```python
from build123d import *

# Parameters (mm, degrees)
SKETCH1_W            = 9.7
SKETCH1_H            = 4.4
BOSS_EXTRUDE1_DEPTH  = 0.42
FILLET1_R            = 1
FILLET2_R            = 1
FILLET3_R            = 1
FILLET4_R            = 1
BOSS_EXTRUDE2_DEPTH  = 0.04
BOSS_EXTRUDE3_DEPTH  = 0.04
BOSS_EXTRUDE4_DEPTH  = 0.04
BOSS_EXTRUDE5_DEPTH  = 0.04
BOSS_EXTRUDE6_DEPTH  = 0.04
BOSS_EXTRUDE7_DEPTH  = 0.04
BOSS_EXTRUDE8_DEPTH  = 0.04
BOSS_EXTRUDE9_DEPTH  = 0.04
BOSS_EXTRUDE10_DEPTH = 0.04
SKETCH11_W           = 0.5
SKETCH11_H           = 1
BOSS_EXTRUDE11_DEPTH = 0.04
SKETCH12_W           = 0.5
SKETCH12_H           = 1
BOSS_EXTRUDE12_DEPTH = 0.04
BOSS_EXTRUDE13_DEPTH = 0.025
HOLE1_D              = 0.3
HOLE2_D              = 0.3
HOLE3_D              = 0.3
CHAMFER1_SIZE        = 0.1
CHAMFER2_SIZE        = 0.05
CHAMFER3_SIZE        = 0.1
CHAMFER4_SIZE        = 0.05
CHAMFER5_SIZE        = 0.1
CHAMFER6_SIZE        = 0.1
CHAMFER7_SIZE        = 0.05
CHAMFER8_SIZE        = 0.05


with BuildPart() as part:
    # Sketch1 → Boss-Extrude1 (new body)
    with BuildSketch(Plane.XY):
        with Locations((4.849999999, 2.20000002)):
            Rectangle(SKETCH1_W, SKETCH1_H)
    extrude(amount=-BOSS_EXTRUDE1_DEPTH)

    # Fillet1
    fillet1_edges = [part.edges().sort_by_distance(p)[0] for p in [
        (-1e-09, 2e-08, -0.21),
    ]]
    fillet(fillet1_edges, radius=FILLET1_R)

    # Fillet2
    fillet2_edges = [part.edges().sort_by_distance(p)[0] for p in [
        (-1e-09, 4.40000002, -0.21),
    ]]
    fillet(fillet2_edges, radius=FILLET2_R)

    # Fillet3
    fillet3_edges = [part.edges().sort_by_distance(p)[0] for p in [
        (9.699999999, 2e-08, -0.21),
    ]]
    fillet(fillet3_edges, radius=FILLET3_R)

    # Fillet4
    fillet4_edges = [part.edges().sort_by_distance(p)[0] for p in [
        (9.699999999, 4.40000002, -0.21),
    ]]
    fillet(fillet4_edges, radius=FILLET4_R)

    # Sketch2 → Boss-Extrude2 (add)
    with BuildSketch(Plane.XY):
        Polygon((3.691646515, 0.405675456), (4.19162877, 0.405675456), (4.19162877, 0.255675455), (5.553515055, 0.255675455), (5.553515055, 0.45000002), (5.853515055, 0.45000002), (5.853515055, 0.05000002), (5.553515055, 0.05000002), (5.553515055, 0.105675455), (4.04162877, 0.105675455), (4.04162877, 0.255675455), (2.69162877, 0.255675455), (2.69162877, 1.625675455), (3.54162877, 1.625675455), (3.54162877, 2.031926109), (2.082430938, 2.031926109), (2.082430938, 2.631926109), (2.432448683, 2.631926109), (2.432448683, 2.97790002), (2.082448683, 2.97790002), (2.082448683, 3.57790002), (2.582448683, 3.57790002), (2.582448683, 2.181926109), (3.691646515, 2.181926109), align=None)
    extrude(amount=BOSS_EXTRUDE2_DEPTH)

    # Sketch3 → Boss-Extrude3 (add)
    with BuildSketch(Plane.XY):
        Polygon((6.356700213, 0.05000002), (6.056700213, 0.05000002), (6.056700213, 0.45000002), (6.356700213, 0.45000002), (6.356700213, 0.25000002), (7.899307242, 0.25000002), (7.899307242, 1.334176783), (7.549307242, 1.334176783), (7.549307242, 2.97790002), (6.425655767, 2.97790002), (6.425655767, 3.97790002), (6.925655767, 3.97790002), (6.925655767, 3.12790002), (7.699307242, 3.12790002), (7.699307242, 1.484176783), (9.269307242, 1.484176783), (9.269307242, 0.484176783), (8.049307242, 0.484176783), (8.049307242, 0.10000002), (6.356700213, 0.10000002), align=None)
    extrude(amount=BOSS_EXTRUDE3_DEPTH)

    # Sketch4 → Boss-Extrude4 (add)
    with BuildSketch(Plane.XY):
        Polygon((1.148250377, 3.831121862), (1.148250377, 3.381121862), (1.398250377, 3.381121862), (1.448250377, 3.431121862), (1.448250377, 3.481121862), (1.548250377, 3.481121862), (1.548250377, 3.381121862), (1.448250377, 3.281121862), (1.048250377, 3.281121862), (1.048250377, 3.931121862), (1.448250377, 3.931121862), (1.548250377, 3.831121862), (1.548250377, 3.731121862), (1.448250377, 3.731121862), (1.448250377, 3.781121862), (1.398250377, 3.831121862), align=None)
    extrude(amount=BOSS_EXTRUDE4_DEPTH)

    # Sketch5 → Boss-Extrude5 (add)
    with BuildSketch(Plane.XY):
        Polygon((0.417468966, 3.281121862), (0.417468966, 3.381121862), (0.467468966, 3.381121862), (0.467468966, 3.831121862), (0.417468966, 3.831121862), (0.417468966, 3.931121862), (0.917468966, 3.931121862), (0.917468966, 3.643621862), (0.817468966, 3.643621862), (0.817468966, 3.831121862), (0.567468966, 3.831121862), (0.567468966, 3.381121862), (0.817468966, 3.381121862), (0.817468966, 3.568621862), (0.917468966, 3.568621862), (0.917468966, 3.281121862), align=None)
    extrude(amount=BOSS_EXTRUDE5_DEPTH)

    # Sketch6 → Boss-Extrude6 (add)
    with BuildSketch(Plane.XY):
        Polygon((5.349999999, 0.385416863), (5.049999999, 0.385416863), (5.049999999, 0.785416863), (5.199999999, 0.785416863), (5.199999999, 1.246726542), (4.349999999, 1.246726542), (4.349999999, 2.616726542), (4.869837207, 2.616726542), (4.869837207, 2.97790002), (4.519837207, 2.97790002), (4.519837207, 3.97790002), (5.019837207, 3.97790002), (5.019837207, 2.616726542), (5.349999999, 2.616726542), align=None)
    extrude(amount=BOSS_EXTRUDE6_DEPTH)

    # Sketch7 → Boss-Extrude7 (add)
    with BuildSketch(Plane.XY):
        Polygon((1.691646515, 1.625675456), (1.691646515, 0.255675456), (0.691646515, 0.255675456), (0.691646515, 2.031926109), (0.241646515, 2.031926109), (0.241646515, 2.631926109), (0.841646515, 2.631926109), (0.841646515, 2.181926109), (1.122933895, 2.181926109), (1.122933895, 2.631926109), (1.622933895, 2.631926109), (1.622933895, 2.031926109), (0.841646515, 2.031926109), (0.841646515, 1.625675456), align=None)
    extrude(amount=BOSS_EXTRUDE7_DEPTH)

    # Sketch8 → Boss-Extrude8 (add)
    with BuildSketch(Plane.XY):
        Polygon((3.54196347, 3.57790002), (3.54196347, 3.12790002), (3.884837207, 3.12790002), (3.884837207, 3.97790002), (4.384819462, 3.97790002), (4.384819462, 2.97790002), (3.041945725, 2.97790002), (3.041945725, 3.57790002), align=None)
    extrude(amount=BOSS_EXTRUDE8_DEPTH)

    # Sketch9 → Boss-Extrude9 (add)
    with BuildSketch(Plane.XY):
        Polygon((6.749999999, 1.088728228), (7.183722976, 1.088728228), (7.183722976, 1.246726542), (6.349999999, 1.246726542), (6.349999999, 2.616726542), (7.349999999, 2.616726542), (7.349999999, 0.488728228), (6.749999999, 0.488728228), align=None)
    extrude(amount=BOSS_EXTRUDE9_DEPTH)

    # Sketch10 → Boss-Extrude10 (add)
    with BuildSketch(Plane.XY):
        Polygon((8.499307242, 3.667992872), (8.053251319, 3.667992872), (8.053251319, 3.484176783), (9.269307242, 3.484176783), (9.269307242, 2.484176783), (7.899307242, 2.484176783), (7.899307242, 4.267992872), (8.499307242, 4.267992872), align=None)
    extrude(amount=BOSS_EXTRUDE10_DEPTH)

    # Sketch11 → Boss-Extrude11 (add)
    with BuildSketch(Plane.XY):
        with Locations((5.404837207, 3.47790002)):
            Rectangle(SKETCH11_W, SKETCH11_H)
    extrude(amount=BOSS_EXTRUDE11_DEPTH)

    # Sketch12 → Boss-Extrude12 (add)
    with BuildSketch(Plane.XY):
        with Locations((6.040655767, 3.47790002)):
            Rectangle(SKETCH12_W, SKETCH12_H)
    extrude(amount=BOSS_EXTRUDE12_DEPTH)

    # Sketch19 → Boss-Extrude13 (add)
    with BuildSketch(Plane(origin=(0, 0, -0.42), x_dir=(-1, 0, 0), z_dir=(0, 0, -1))):
        with BuildLine():
            Line((-0.999999999, 4.30000002), (-8.699999999, 4.30000002))
            ThreePointArc((-8.699999999, 4.30000002), (-9.336396102, 4.036396123), (-9.599999999, 3.40000002))
            Line((-9.599999999, 3.40000002), (-9.599999999, 1.00000002))
            ThreePointArc((-9.599999999, 1.00000002), (-9.336396102, 0.363603917), (-8.699999999, 0.10000002))
            Line((-8.699999999, 0.10000002), (-0.999999999, 0.10000002))
            ThreePointArc((-0.999999999, 0.10000002), (-0.363603896, 0.363603917), (-0.099999999, 1.00000002))
            Line((-0.099999999, 1.00000002), (-0.099999999, 3.40000002))
            ThreePointArc((-0.099999999, 3.40000002), (-0.363603896, 4.036396123), (-0.999999999, 4.30000002))
        make_face()
    extrude(amount=BOSS_EXTRUDE13_DEPTH)

    # Hole1 (through all)
    with Locations(Plane.XY.offset(0.04)):
        with Locations((8.199307242, 3.967992872)):
            Hole(HOLE1_D / 2)

    # Hole2 (through all)
    with Locations(Plane.XY.offset(0.04)):
        with Locations((7.049999999, 0.788728228)):
            Hole(HOLE2_D / 2)

    # Hole3 (through all)
    with Locations(Plane.XY.offset(0.04)):
        with Locations((0.541646515, 2.331926109)):
            Hole(HOLE3_D / 2)

    # Chamfer1
    chamfer1_edges = [part.edges().sort_by_distance(p)[0] for p in [
        (0.917468966, 3.931121862, 0.02),
    ]]
    chamfer(chamfer1_edges, length=CHAMFER1_SIZE)

    # Chamfer2
    chamfer2_edges = [part.edges().sort_by_distance(p)[0] for p in [
        (1.148250377, 3.831121862, 0.02),
    ]]
    chamfer(chamfer2_edges, length=CHAMFER2_SIZE)

    # Chamfer3
    chamfer3_edges = [part.edges().sort_by_distance(p)[0] for p in [
        (0.917468966, 3.281121862, 0.02),
    ]]
    chamfer(chamfer3_edges, length=CHAMFER3_SIZE)

    # Chamfer4
    chamfer4_edges = [part.edges().sort_by_distance(p)[0] for p in [
        (0.817468966, 3.831121862, 0.02),
    ]]
    chamfer(chamfer4_edges, length=CHAMFER4_SIZE)

    # Chamfer5
    chamfer5_edges = [part.edges().sort_by_distance(p)[0] for p in [
        (1.048250377, 3.281121862, 0.02),
    ]]
    chamfer(chamfer5_edges, length=CHAMFER5_SIZE)

    # Chamfer6
    chamfer6_edges = [part.edges().sort_by_distance(p)[0] for p in [
        (1.048250377, 3.931121862, 0.02),
    ]]
    chamfer(chamfer6_edges, length=CHAMFER6_SIZE)

    # Chamfer7
    chamfer7_edges = [part.edges().sort_by_distance(p)[0] for p in [
        (1.148250377, 3.381121862, 0.02),
    ]]
    chamfer(chamfer7_edges, length=CHAMFER7_SIZE)

    # Chamfer8
    chamfer8_edges = [part.edges().sort_by_distance(p)[0] for p in [
        (0.817468966, 3.381121862, 0.02),
    ]]
    chamfer(chamfer8_edges, length=CHAMFER8_SIZE)


solid = part.part
```
Build history of the part. All positions in model axes, mm. Give positions to 0.01 mm unless a question says otherwise; leave off trailing zeros. Loops run counter-clockwise (first coordinate to the right, second up) from the corner with the lowest first, then second, coordinate; pieces in that order, holes last.
1) Probe line 1 along Y through (x, z) = (7.05, -0.05); line 2 along Z through (x, y) = (2.75, 1.7) (3 decimals); line 3 along X through (y, z) = (0.75, -0.1). List the from-to ranges inside material, lowest first.
Values follow:
line 1: y = 0 to 0.64, 0.94 to 4.4
line 2: z = -0.445 to 0
line 3: x = 0.03 to 6.91, 7.19 to 9.67
2) Band-saw the part on A-A on x = 7.05. List the corners of the cut face in (y, z) (3 decimals), then the cut area to 3 significant figures.
Values follow:
outline: (0, -0.42) - (0.1, -0.42) - (0.1, -0.445) - (0.639, -0.445) - (0.639, 0.04) - (0.489, 0.04) - (0.489, 0) - (0.25, 0) - (0.25, 0.04) - (0.1, 0.04) - (0.1, 0) - (0, 0) - close; (0.939, -0.445) - (4.3, -0.445) - (4.3, -0.42) - (4.4, -0.42) - (4.4, 0) - (3.128, 0) - (3.128, 0.04) - (2.978, 0.04) - (2.978, 0) - (2.617, 0) - (2.617, 0.04) - (1.247, 0.04) - (1.247, 0) - (1.089, 0) - (1.089, 0.04) - (0.939, 0.04) - close
area: 1.90 mm2
3) Band-saw the part on C-C on z = -0.3. List the corners of the cut face in (x, y), then the cut area to 3 significant figures.
Values follow:
outline: (0, 1) arc R1 ccw to (1, 0) - (8.7, 0) arc R1 ccw to (9.7, 1) - (9.7, 3.4) arc R1 ccw to (8.7, 4.4) - (1, 4.4) arc R1 ccw to (0, 3.4) - close; hole circle Ø0.3 at (0.54, 2.33); hole circle Ø0.3 at (7.05, 0.79); hole circle Ø0.3 at (8.2, 3.97)
area: 41.6 mm2
4) Two-plate mould, pull along X, no slides. Class faces 1 (the face through (7, 2, 0.04)), 2 (the face through (4, 2, 0)), 3 (the face through (0.285, 4.099, -0.213)), 4 (the face through (9.415, 4.099, -0.213)): released by +X, released by -X, zero draft, split by the parting line, or undercut.
Values follow:
face 1: zero draft
face 2: undercut
face 3: released by -X
face 4: released by +X
5) Band-saw the part on B-B on y = 1.9. List the corners of the cut face in (x, z) (3 decimals).
Values follow:
outline: (0, -0.42) - (0.1, -0.42) - (0.1, -0.445) - (9.6, -0.445) - (9.6, -0.42) - (9.7, -0.42) - (9.7, 0) - (7.699, 0) - (7.699, 0.04) - (7.549, 0.04) - (7.549, 0) - (7.35, 0) - (7.35, 0.04) - (6.35, 0.04) - (6.35, 0) - (5.35, 0) - (5.35, 0.04) - (4.35, 0.04) - (4.35, 0) - (3.692, 0) - (3.692, 0.04) - (3.542, 0.04) - (3.542, 0) - (0.842, 0) - (0.842, 0.04) - (0.692, 0.04) - (0.692, 0) - (0, 0) - close
6) Drop a flat-ended pin along its axis: P1, Ø2, axis at x = 2, y = 1.5, coming from the +Z side. Give the stop position or say it passes through.
Values follow:
P1: stops at z = 0.04
